Job drawing, mm, ordinate dimensions from the low corner. One solid piece. A direction names the side the tool comes from. Round coordinates to 2 decimals unless told otherwise and drop trailing zeros. Loops run counter-clockwise (first coordinate to the right, second up) from the corner with the lowest first, then second, coordinate; pieces in that order, holes last.
1) Band-saw the part on C-C, the plane x = 29. Write the cut outline in (y, z).
2) 3-axis set-ups, long thin cutter, end or side, ignore diameter. For the marked faces 1, 2 and 3: which of +Z, -Z, +X, -X, +Y, -Y reach the whole face in a straight line?
3) Band-saw the part on B-B, the plane z = 5. Write the cut outline in (x, y), then the cut area to 3 significant figures.
4) Drop flat-ended pins along their axis: P1, Ø2.5, axis at x = 4.5, y = 13.5, coming from the +Z side; P2, Ø1.8, axis at y = 2.5, z = 8.5, coming from the -X side; P3, Ø4, axis at x = 27.5, y = 12, coming from the +Z side; P4, Ø5, axis at y = 4.5, z = 29.5, coming from the -X side. Give the stop position or say it passes through.
5) Mould opens along X. For the marked faces 4, 5 and 6 say: +X half, -X half, draft (parallel to the pull), parting line (faces both ways), or undercut.
6) Band-saw the part on A-A, the plane x = 63. Write the cut outline in (y, z).
7) Band-saw the part on D-D, the plane z = 36. Write the cut outline in (x, y).
8) Probe line 1 (Z direction, x = 63, y = 2.1); line 2 (X direction, y = 0.8, z = 5); line 3 (X direction, y = 2.5, z = 19) (1 decimal). List the from-to ranges inside material, lowest first.
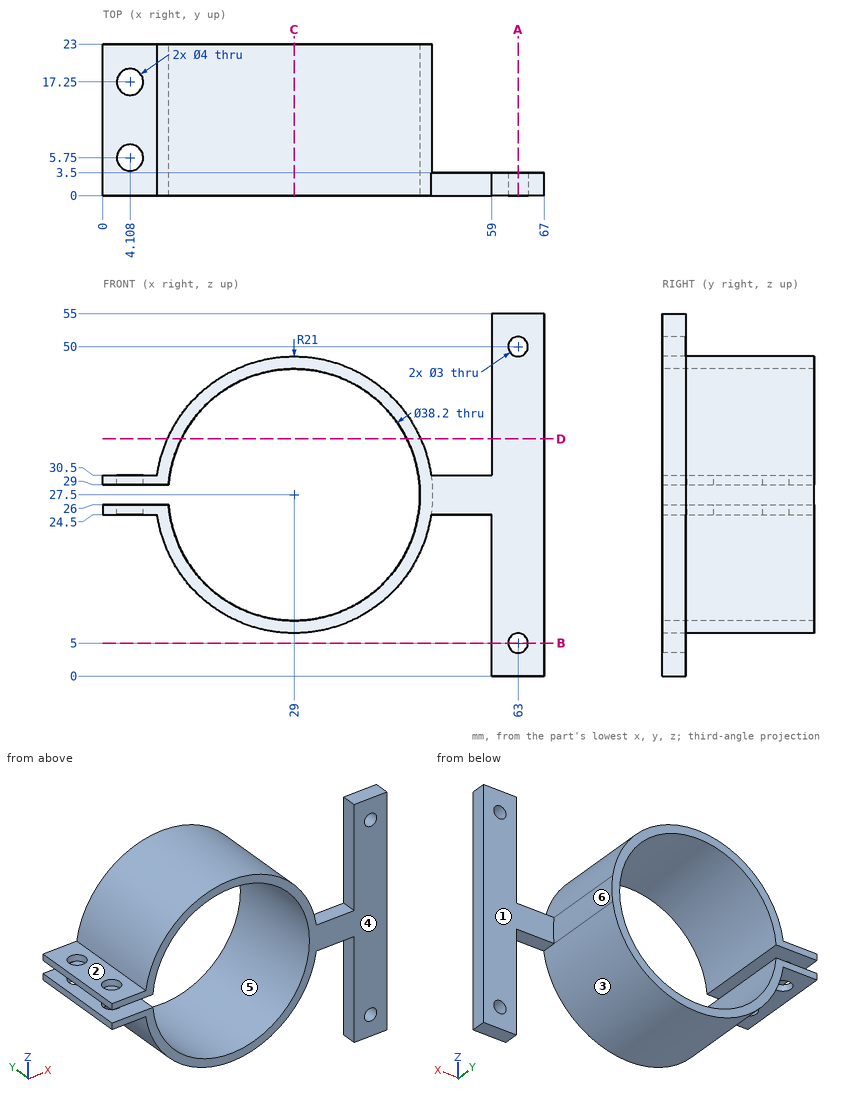
Reported:
1. outline: (0, 6.5) - (23, 6.5) - (23, 8.4) - (0, 8.4) - close; (0, 46.6) - (23, 46.6) - (23, 48.5) - (0, 48.5) - close
2. face 1: +Z, -Z, +X, +Y
2. face 2: +Z, -X, +Y, -Y
2. face 3: -Z, +Y, -Y
3. outline: (59, 0) - (61.5, 0) - (61.5, 3.5) - (59, 3.5) - close; (64.5, 0) - (67, 0) - (67, 3.5) - (64.5, 3.5) - close
3. area: 17.5 mm2
4. P1: stops at z = 30.5
4. P2: stops at x = 18.35
4. P3: stops at z = 48.5
4. P4: stops at x = 0
5. face 4: draft
5. face 5: undercut
5. face 6: +X half
6. outline: (0, 0) - (3.5, 0) - (3.5, 3.5) - (0, 3.5) - close; (0, 6.5) - (3.5, 6.5) - (3.5, 48.5) - (0, 48.5) - close; (0, 51.5) - (3.5, 51.5) - (3.5, 55) - (0, 55) - close
7. outline: (9.8, 0) - (11.9, 0) - (11.9, 23) - (9.8, 23) - close; (46.1, 0) - (48.2, 0) - (48.2, 23) - (46.1, 23) - close; (59, 0) - (67, 0) - (67, 3.5) - (59, 3.5) - close
8. line 1: z = 0 to 3.5, 6.5 to 48.5, 51.5 to 55
8. line 2: x = 59 to 61.5, 64.5 to 67
8. line 3: x = 9.8 to 11.9, 46.1 to 48.2, 59 to 67
